For this review, take the finished solid that the model builds, in its own axes (mm). A direction names the side the tool comes from. Coordinates: 2 decimals unless noted, no trailing zeros. Write each loop counter-clockwise with the first axis right and the second up, starting at its lowest first coordinate (ties: lowest second). Pieces come first, ordered by that corner, then holes.
1) Insertion check: P1, Ø9.5, axis at y = 9, z = -5, coming from the +X side; P2, Ø4, axis at y = 43, z = -40, coming from the -X side. Each pin has a flat end and moves straight along its axis. Give the tip position at first contact, or say it passes through.
2) To check wall thickness, follow line 1 along Y through (x, z) = (119, 24.5); line 2 along X through (y, z) = (7.5, 7); line 3 along Z through (x, y) = (50.5, 15.5). State the ranges of each line that lie inside material, in increasing order.
3) We need section C-C on z = 109. Write out the cut boundary in (x, y), then the cut area to 3 significant figures.
4) For faces 1 (the face through (-39.84, 83.439, -68.294)), 2 (the face through (25.4, 9, 0)), 3 (the face through (-12.91, 53.44, -73.16)), list the 3-axis set-ups (+Z, -Z, +X, -X, +Y, -Y) from which the entire face can be reached by the end or side of a thin tool; tool diameter is ignored.
5) Mouldability with a two-part tool opening along X and no side actions: class faces 4 (the face through (-59.06, 67.55, -51.494)), 5 (the face through (12.878, 9.392, 21.894)), 6 (the face through (-28.27, 81.66, -49.67)) as pulls with the +X half, pulls with the -X half, needs draft (parallel to the pull), parting line crosses it, or undercut.
6) We need section D-D on y = 41.5. Write out the cut boundary in (x, z).
7) We need section A-A on z = 21.5. Write out the cut boundary in (x, y), then the cut area to 3 significant figures.
8) We need section B-B on x = -42. Write out the cut boundary in (y, z).
from build123d import *

# Parameters (mm, degrees)
BOSS_EXTRUDE1_DEPTH = 19.05
BOSS_EXTRUDE2_DEPTH = 127
CUT_EXTRUDE1_DEPTH  = 282.074619797


with BuildPart() as part:
    # Sketch2 → Boss-Extrude1 (new body)
    # profile 1 of 5: a face of its own
    with BuildSketch(Plane(origin=(0, 0, 0), x_dir=(1, 0, 0), z_dir=(0, 1, 0))):
        with BuildLine():
            ThreePointArc((-149.056021348, 31.75), (-151.561699735, 15.962805935), (-152.4, 0))
            Line((-152.4, 0), (-139.7, 0))
            Line((-139.7, 0), (-139.7, 31.75))
            Line((-139.7, 31.75), (-149.056021348, 31.75))
        make_face()
    # profile 2 of 5: a face of its own
    with BuildSketch(Plane(origin=(0, 0, 0), x_dir=(1, 0, 0), z_dir=(0, 1, 0))):
        with BuildLine():
            ThreePointArc((0, 152.4), (-15.962805935, 151.561699735), (-31.75, 149.056021348))
            Line((-31.75, 149.056021348), (-31.75, 139.7))
            Line((-31.75, 139.7), (0, 139.7))
            Line((0, 139.7), (0, 152.4))
        make_face()
    # profile 3 of 5: a face of its own
    with BuildSketch(Plane(origin=(0, 0, 0), x_dir=(1, 0, 0), z_dir=(0, 1, 0))):
        with BuildLine():
            Line((139.7, -31.75), (149.056021348, -31.75))
            ThreePointArc((149.056021348, -31.75), (151.561699735, -15.962805935), (152.4, 0))
            Line((152.4, 0), (139.7, 0))
            Line((139.7, 0), (139.7, -31.75))
        make_face()
    # profile 4 of 5: a face of its own
    with BuildSketch(Plane(origin=(0, 0, 0), x_dir=(1, 0, 0), z_dir=(0, 1, 0))):
        with BuildLine():
            Line((0, -139.7), (0, -152.4))
            ThreePointArc((0, -152.4), (15.962805935, -151.561699735), (31.75, -149.056021348))
            Line((31.75, -149.056021348), (31.75, -139.7))
            Line((31.75, -139.7), (0, -139.7))
        make_face()
    # profile 5 of 5: a face of its own
    with BuildSketch(Plane(origin=(0, 0, 0), x_dir=(1, 0, 0), z_dir=(0, 1, 0))):
        with BuildLine():
            Line((-139.7, 0), (-152.4, 0))
            ThreePointArc((-152.4, 0), (-107.763073453, -107.763073453), (0, -152.4))
            Line((0, -152.4), (0, -139.7))
            Line((0, -139.7), (31.75, -139.7))
            Line((31.75, -139.7), (31.75, -149.056021348))
            ThreePointArc((31.75, -149.056021348), (107.763073453, -107.763073453), (149.056021348, -31.75))
            Line((149.056021348, -31.75), (139.7, -31.75))
            Line((139.7, -31.75), (139.7, 0))
            Line((139.7, 0), (152.4, 0))
            ThreePointArc((152.4, 0), (107.763073453, 107.763073453), (0, 152.4))
            Line((0, 152.4), (0, 139.7))
            Line((0, 139.7), (-31.75, 139.7))
            Line((-31.75, 139.7), (-31.75, 149.056021348))
            ThreePointArc((-31.75, 149.056021348), (-107.763073453, 107.763073453), (-149.056021348, 31.75))
            Line((-149.056021348, 31.75), (-139.7, 31.75))
            Line((-139.7, 31.75), (-139.7, 0))
        make_face()
        Polygon((-25.4, 14.664696837), (0, 29.329393675), (25.4, 14.664696837), (25.4, -14.664696837), (0, -29.329393675), (-25.4, -14.664696837), align=None, mode=Mode.SUBTRACT)
    extrude(amount=BOSS_EXTRUDE1_DEPTH)

    # Sketch3 → Boss-Extrude2 (add)
    with BuildSketch(Plane(origin=(0, 19.05, 0), x_dir=(1, 0, 0), z_dir=(0, 1, 0))):
        Polygon((-50.572045256, 36.793351826), (-72.797045256, 75.288181024), (-28.802954744, 100.688181024), (-6.577954744, 62.193351826), align=None)
    extrude(amount=BOSS_EXTRUDE2_DEPTH)

    # Sketch5 → Cut-Extrude1 (cut, through all)
    with BuildSketch(Plane(origin=(-21.997045256, 0, 12.7), x_dir=(0.5, 0, 0.8660254037844386), z_dir=(-0.8660254037844387, 0, 0.5000000000000001))):
        Polygon((-101.6, 19.05), (-101.6, 146.05), (-57.15, 146.05), align=None)
    extrude(amount=-CUT_EXTRUDE1_DEPTH, mode=Mode.SUBTRACT)


solid = part.part
Result:
1. P1: stops at x = 152.4
1. P2: stops at x = -53.58
2. line 1: y = 0 to 19.05
2. line 2: x = -152.24 to -25.4, 25.4 to 152.24
2. line 3: z = -143.79 to 143.79
3. outline: (-106.51, 0) - (106.51, 0) - (106.51, 19.05) - (-106.51, 19.05) - close
3. area: 4,060 mm2
4. face 1: -Z, -X, +Y
4. face 2: +Y, -Y
4. face 3: -Z, +X, +Y
5. face 4: pulls with the -X half
5. face 5: undercut
5. face 6: pulls with the +X half
6. outline: (-68.87, -68.48) - (-24.87, -93.88) - (-6.58, -62.19) - (-50.57, -36.79) - close
7. outline: (-150.88, 0) - (-13.56, 0) - (-13.56, 19.05) - (-150.88, 19.05) - close; (13.56, 0) - (150.88, 0) - (150.88, 19.05) - (13.56, 19.05) - close
7. area: 5,230 mm2
8. outline: (0, -146.5) - (19.05, -146.5) - (19.05, -93.07) - (146.05, -41.74) - (19.05, -41.74) - (19.05, 146.5) - (0, 146.5) - close
